Geometry: see drawing. Coordinates: mm, zero at the bounding-box minimum. A direction names the side the tool comes from. Give positions to 0.01 mm unless a question says otherwise; leave off trailing zeros. Order: outer loops, then holes, each group sorted by start corner. A loop starts at its lowest first (then second) coordinate and runs counter-clockwise, first axis right, second up. Notation, with made-up numbers: (3, 84) -> (34, 84) arc R21 cw to (34, 115) -> close; hole circle Ø1 at (14.5, 4). An arc over 180 degrees is marked (long way). One line per item, written item: value. Start each with the question number.
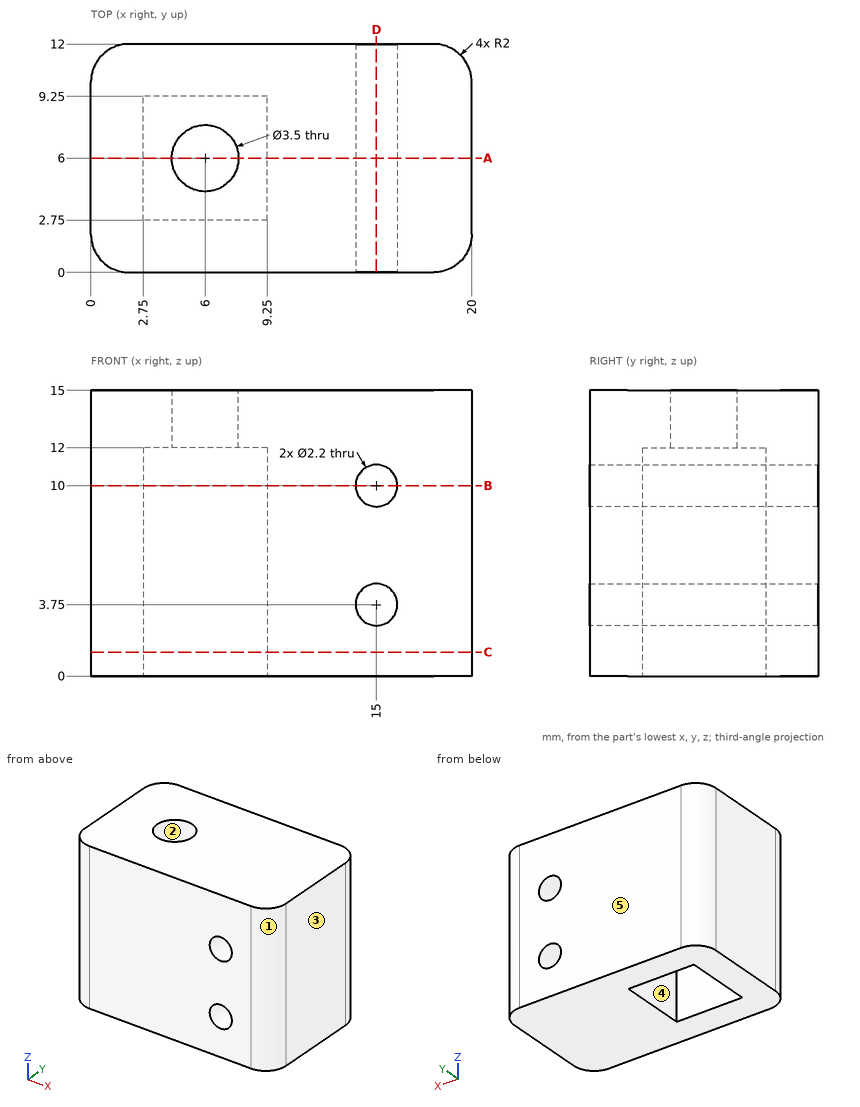
1. Draft query along Y for the marked faces 1, 2 and 3. Return one class per face: pulls with the +Y half, pulls with the -Y half, needs draft (parallel to the pull), parting line crosses it, or undercut.
2. Access query for the marked faces 4 and 5. Directions: +Z, -Z, +X, -X, +Y, -Y. A direction counts if a zero-diameter tool reaches every point of the face in a straight line with its end or side. Return the directions, or none.
3. Cut plane A-A, the plane y = 6. Return loops of the section in (x, z), then the cut area to 3 significant figures.
4. Cut plane C-C, the plane z = 1.25. Return loops of the section in (x, y).
5. Pin query (flat end, axial travel): P1, Ø8, axis at x = 4.5, z = 10, coming from the -Y side; P2, Ø4, axis at x = 6, y = 6, coming from the -Z side. Return the tip coordinate at first contact, or that it passes through.
6. Cut plane B-B, the plane z = 10. Return loops of the section in (x, y).
7. Material intervals for L1, parallel to Z at x = 15, y = 8.75; L2, parallel to X at y = 6.75, z = 3.75; L3, parallel to Y at x = 5, z = 9, sorted ascending. Write a range as [from, to].
8. Cut plane D-D, the plane x = 15. Return loops of the section in (y, z).
Answers follow:
1. face 1: pulls with the -Y half
1. face 2: undercut
1. face 3: needs draft
2. face 4: -Z
2. face 5: +Z, -Z, +X, -X, +Y
3. outline: (0, 0) -> (2.75, 0) -> (2.75, 12) -> (4.25, 12) -> (4.25, 15) -> (0, 15) -> close; (7.75, 12) -> (9.25, 12) -> (9.25, 0) -> (20, 0) -> (20, 15) -> (7.75, 15) -> close; hole circle Ø2.2 at (15, 3.75); hole circle Ø2.2 at (15, 10)
3. area: 204 mm²
4. outline: (0, 2) arc R2 ccw to (2, 0) -> (18, 0) arc R2 ccw to (20, 2) -> (20, 10) arc R2 ccw to (18, 12) -> (2, 12) arc R2 ccw to (0, 10) -> close; hole (2.75, 2.75) -> (9.25, 2.75) -> (9.25, 9.25) -> (2.75, 9.25) -> close
5. P1: stops at y = 0
5. P2: stops at z = 12
6. outline: (0, 2) arc R2 ccw to (2, 0) -> (13.9, 0) -> (13.9, 12) -> (2, 12) arc R2 ccw to (0, 10) -> close; (16.1, 0) -> (18, 0) arc R2 ccw to (20, 2) -> (20, 10) arc R2 ccw to (18, 12) -> (16.1, 12) -> close; hole (2.75, 2.75) -> (9.25, 2.75) -> (9.25, 9.25) -> (2.75, 9.25) -> close
7. L1: z = [0, 2.65], [4.85, 8.9], [11.1, 15]
7. L2: x = [0, 2.75], [9.25, 13.9], [16.1, 20]
7. L3: y = [0, 2.75], [9.25, 12]
8. outline: (0, 0) -> (12, 0) -> (12, 2.65) -> (0, 2.65) -> close; (0, 4.85) -> (12, 4.85) -> (12, 8.9) -> (0, 8.9) -> close; (0, 11.1) -> (12, 11.1) -> (12, 15) -> (0, 15) -> close
